Geometry: see drawing. Coordinates: mm, zero at the bounding-box minimum. A direction names the side the tool comes from. Round coordinates to 2 decimals unless told otherwise and drop trailing zeros. Write each loop counter-clockwise with the first axis right and the second up, starting at its lowest first coordinate (ties: lowest second). Pieces come first, ordered by that corner, then holes. Notation, with made-up numbers: (55, -4) -> (62, -4) arc R27 ccw to (62, 22) -> close; hole circle Ø5 at (45.25, 83.5). An arc over 180 degrees is marked (long way). Write item = value, one per line.
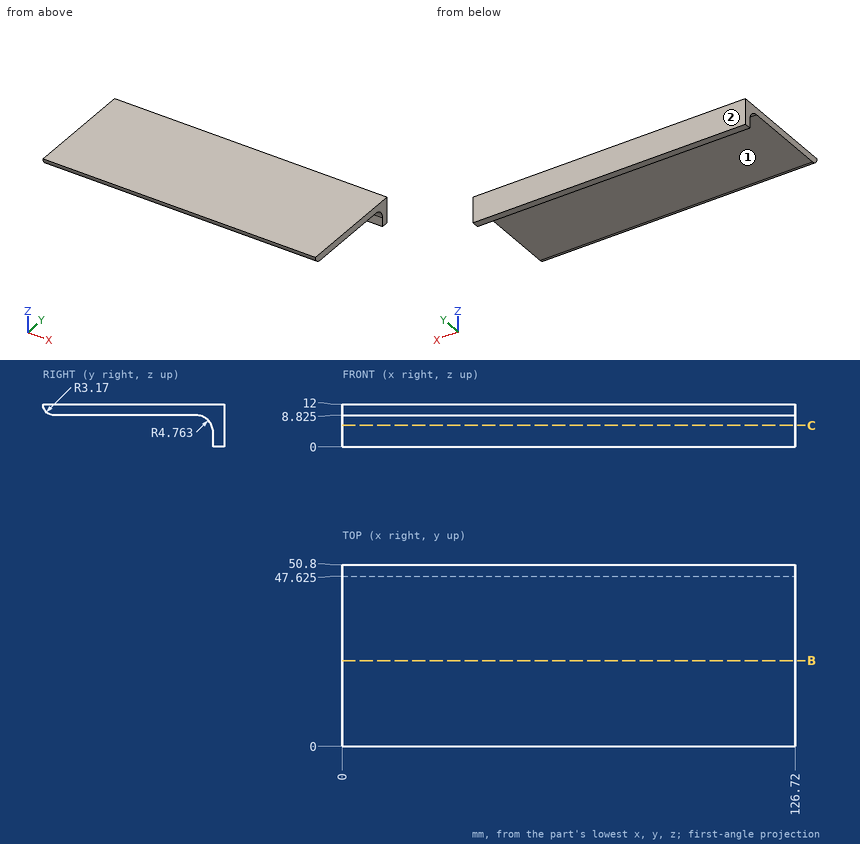
1) Line query: L1, parallel to Y at x = 86.5, z = 2 (1 decimal); L2, parallel to Z at x = 115.5, y = 6 (1 decimal); L3, parallel to Y at x = 42, z = 7.25. Output: solid intervals per line, ascending. Write a range as from..to.
Solutions:
L1 = 47.6..50.8
L2 = 8.8..12
L3 = 46.4..50.8
2) Access query for the marked faces 1 and 2. Directions: +Z, -Z, +X, -X, +Y, -Y. A direction counts if a zero-diameter tool reaches every point of the face in a straight line with its end or side. Return the directions, or none.
Solutions:
face_1 = -Z, +X, -X, -Y
face_2 = +Z, -Z, +X, -X, +Y
3) Cut plane C-C (z = 6). Return the cut outline in (x, y).
Solutions:
outline = (0, 47.21) -> (126.72, 47.21) -> (126.72, 50.8) -> (0, 50.8) -> close
4) Cut plane B-B (y = 24). Return the cut outline in (x, z) (1 decimal).
Solutions:
outline = (0, 8.8) -> (126.7, 8.8) -> (126.7, 12) -> (0, 12) -> close
5) First-contact query: P1, Ø5, axis at x = 24.5, y = 25, coming from the -Z side (1 decimal); P2, Ø1.5, axis at x = 39.5, z = 6.5, coming from the -Y side; P3, Ø1.2, axis at x = 80, z = 3, coming from the -Y side (1 decimal); P4, Ø4, axis at y = 8, z = 6, coming from the +X side. Flat tips, straight axial feed; report the tip coordinate or a pass-through.
Solutions:
P1 = 8.8
P2 = 46.4
P3 = 47.6
P4 = through
